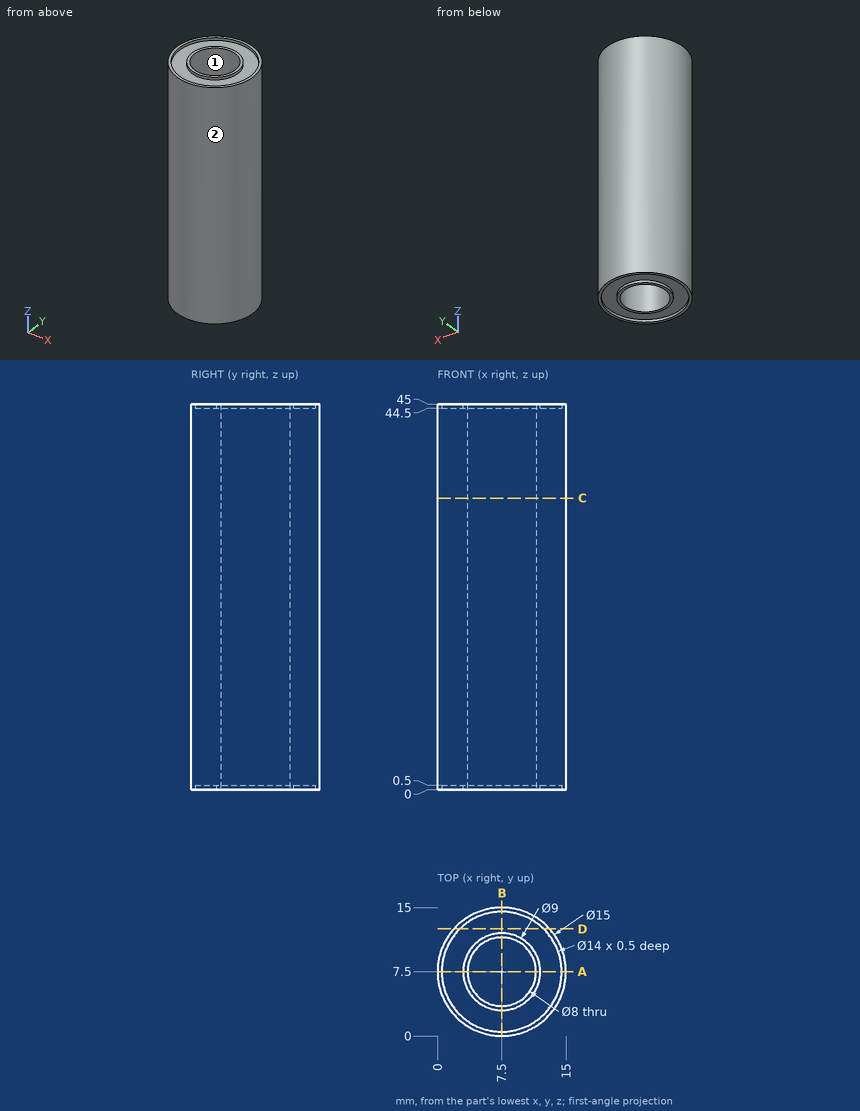
Here's the drawing with two shaded views (mm, measured from the low corner). I have some questions. Give positions to 0.01 mm unless a question says otherwise; leave off trailing zeros. Loops run counter-clockwise (first coordinate to the right, second up) from the corner with the lowest first, then second, coordinate; pieces in that order, holes last. Notation, with made-up numbers: M -2,33 L 52,33 A37 ccw 52,70 Z; hole C 39.25,37 d9. An arc over 180 degrees is marked long. Answer in a Markdown table with one row per item.
1. Suppose I cut it at C-C on z = 34. Write out the boundary of the cut face in (x, y).
Taken from the geometry:
| item | result |
|---|---|
| outline | C 7.5,7.5 d15; hole C 7.5,7.5 d8 |
2. Thinking about a two-plate mould opening in Y: for the marked faces 1 and 2, which applies, released by +Y, released by -Y, zero draft, split by the parting line, or undercut?
Taken from the geometry:
| item | result |
|---|---|
| face 1 | undercut |
| face 2 | split by the parting line |
3. Suppose I cut it at A-A on y = 7.5. Write out the boundary of the cut face in (x, z), plus the area to 3 significant figures.
Taken from the geometry:
| item | result |
|---|---|
| outline | M 0,0 L 0.5,0 L 0.5,0.5 L 3,0.5 L 3,0 L 3.5,0 L 3.5,45 L 3,45 L 3,44.5 L 0.5,44.5 L 0.5,45 L 0,45 Z; M 11.5,0 L 12,0 L 12,0.5 L 14.5,0.5 L 14.5,0 L 15,0 L 15,45 L 14.5,45 L 14.5,44.5 L 12,44.5 L 12,45 L 11.5,45 Z |
| area | 310 mm² |
4. For pin 1 Ø5 at (y, z) = (2.5, 27.5) entering from -X; pin 2 Ø1.5 at (x, z) = (12, 19.5) entering from +Y; pin 3 Ø5 at (x, y) = (10.5, 3.5) entering from +Z; pin 4 Ø1 at (x, y) = (6.5, 12.5) entering from +Z, each with a flat end and sliding along its axis, tell me the tip position at first contact or that it passes through.
Taken from the geometry:
| item | result |
|---|---|
| pin 1 | stops at x = 0.43 |
| pin 2 | stops at y = 14 |
| pin 3 | stops at z = 45 |
| pin 4 | stops at z = 44.5 |
5. Suppose I cut it at D-D on y = 12.5. Write out the boundary of the cut face in (x, z).
Taken from the geometry:
| item | result |
|---|---|
| outline | M 1.91,0 L 2.6,0 L 2.6,0.5 L 12.4,0.5 L 12.4,0 L 13.09,0 L 13.09,45 L 12.4,45 L 12.4,44.5 L 2.6,44.5 L 2.6,45 L 1.91,45 Z |
6. If I drill on line 1 along Y through (x, z) = (7.5, 0.2); line 2 along Y through (x, z) = (7.5, 35); line 3 along Z through (x, y) = (9.5, 13.5), over which ranges is the centre line in solid material (lowest first)?
Taken from the geometry:
| item | result |
|---|---|
| line 1 | y = 0 to 0.5, 3 to 3.5, 11.5 to 12, 14.5 to 15 |
| line 2 | y = 0 to 3.5, 11.5 to 15 |
| line 3 | z = 0.5 to 44.5 |
